For this review, take the finished solid that the model builds, in its own axes (mm). Round coordinates to 2 decimals unless told otherwise and drop trailing zeros. Loops run counter-clockwise (first coordinate to the right, second up) from the corner with the lowest first, then second, coordinate; pieces in that order, holes last. Notation, with made-up numbers: (75.5, -1) -> (107.5, -1) arc R10 ccw to (107.5, 6) -> close; hole circle Ø5 at (-15.5, 34.5). An arc over 180 degrees is marked (long way). Write each question's results on one line, items separated by ' | '.
```python
from build123d import *

# Parameters (mm, degrees)
SKETCH1_W           = 47.625
SKETCH1_H           = 152.4
SKETCH1_R           = 14.2875
BOSS_EXTRUDE1_DEPTH = 6.35
CUT_EXTRUDE1_DEPTH  = 81.086188923
FILLET1_R           = 2.54


with BuildPart() as part:
    # Sketch1 → Boss-Extrude1 (new body)
    with BuildSketch(Plane(origin=(0, 0, 0), x_dir=(1, 0, 0), z_dir=(0, 1, 0))):
        Rectangle(SKETCH1_W, SKETCH1_H)
        with Locations(Location((0, 38.1, 0), (0, 0, 270))):
            Circle(SKETCH1_R, mode=Mode.SUBTRACT)
        with Locations(Location((0, -46.99, 0), (0, 0, 270))):
            Circle(SKETCH1_R, mode=Mode.SUBTRACT)
    extrude(amount=BOSS_EXTRUDE1_DEPTH)

    # Sketch2 → Cut-Extrude1 (cut, through all)
    with BuildSketch(Plane(origin=(0, 6.35, 0), x_dir=(1, 0, 0), z_dir=(0, 1, 0))):
        with BuildLine():
            ThreePointArc((23.8125, -46.99), (0, -70.8025), (-23.8125, -46.99))
            Line((-23.8125, -46.99), (-23.8125, -76.2))
            Line((-23.8125, -76.2), (23.8125, -76.2))
            Line((23.8125, -76.2), (23.8125, -46.99))
        make_face()
        with BuildLine():
            Line((-17.4625, 69.85), (-17.4625, 54.289386956))
            ThreePointArc((-17.4625, 54.289386956), (-10.963825458, 59.238346377), (-3.175, 61.699884136))
            Line((-3.175, 61.699884136), (-3.175, 69.85))
            Line((-3.175, 69.85), (-17.4625, 69.85))
        make_face()
        with BuildLine():
            ThreePointArc((-3.175, 14.500115864), (-10.963825458, 16.961653623), (-17.4625, 21.910613044))
            Line((-17.4625, 21.910613044), (-17.4625, -30.800613044))
            ThreePointArc((-17.4625, -30.800613044), (-10.963825458, -25.851653623), (-3.175, -23.390115864))
            Line((-3.175, -23.390115864), (-3.175, 14.500115864))
        make_face()
        with BuildLine():
            ThreePointArc((3.175, 61.699884136), (10.963825458, 59.238346377), (17.4625, 54.289386956))
            Line((17.4625, 54.289386956), (17.4625, 69.85))
            Line((17.4625, 69.85), (3.175, 69.85))
            Line((3.175, 69.85), (3.175, 61.699884136))
        make_face()
        with BuildLine():
            Line((17.4625, -30.800613044), (17.4625, 21.910613044))
            ThreePointArc((17.4625, 21.910613044), (10.963825458, 16.961653623), (3.175, 14.500115864))
            Line((3.175, 14.500115864), (3.175, -23.390115864))
            ThreePointArc((3.175, -23.390115864), (10.963825458, -25.851653623), (17.4625, -30.800613044))
        make_face()
    extrude(amount=-CUT_EXTRUDE1_DEPTH, mode=Mode.SUBTRACT)

    # Fillet1
    fillet1_edges = [part.edges().sort_by_distance(p)[0] for p in [
        (17.4625, 3.175, 30.800613044),
        (3.175, 3.175, 23.390115864),
        (3.175, 3.175, -14.500115864),
        (17.4625, 3.175, -21.910613044),
        (-3.175, 3.175, 23.390115864),
        (-17.4625, 3.175, 30.800613044),
        (-17.4625, 3.175, -21.910613044),
        (-3.175, 3.175, -14.500115864),
        (-3.175, 3.175, -61.699884136),
        (-17.4625, 3.175, -54.289386956),
        (-17.4625, 3.175, -69.85),
        (-3.175, 3.175, -69.85),
        (17.4625, 3.175, -54.289386956),
        (3.175, 3.175, -61.699884136),
        (3.175, 3.175, -69.85),
        (17.4625, 3.175, -69.85),
    ]]
    fillet(fillet1_edges, radius=FILLET1_R)


solid = part.part
```
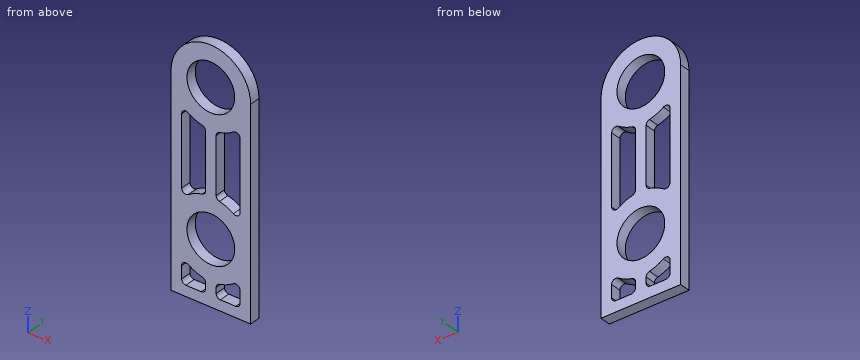
1. Consider section A-A (x = 0). State the section outline as (y, z) points.
Values found:
outline: (0, -76.2) -> (6.35, -76.2) -> (6.35, -52.39) -> (0, -52.39) -> close; (0, -23.81) -> (6.35, -23.81) -> (6.35, 32.7) -> (0, 32.7) -> close; (0, 61.28) -> (6.35, 61.28) -> (6.35, 70.8) -> (0, 70.8) -> close
2. Consider section B-B (z = -38.1). State the section outline as (x, y) points, plus the area to 3 significant figures.
Values found:
outline: (-23.81, 0) -> (-14.29, 0) -> (-14.29, 6.35) -> (-23.81, 6.35) -> close; (14.29, 0) -> (23.81, 0) -> (23.81, 6.35) -> (14.29, 6.35) -> close | area: 121 mm2
3. To check wall thickness, follow probe 1 along X at (y, z) = (4, 6) (1 decimal); probe 2 along Z at (x, y) = (12, 4); probe 3 along Z at (x, y) = (-4.5, 2.5). State the ranges of each line that lie inside material, in increasing order.
Values found:
probe 1: x = -23.8 to -17.5, -3.2 to 3.2, 17.5 to 23.8 | probe 2: z = -76.2 to -69.85, -58.67 to -45.85, -30.35 to -17.53, 26.42 to 39.24, 54.74 to 67.56 | probe 3: z = -76.2 to -69.54, -61.59 to -51.66, -24.54 to -14.61, 23.5 to 33.43, 60.55 to 70.37
4. Consider section D-D (x = 7.5). State the section outline as (y, z) points.
Values found:
outline: (0, -76.2) -> (6.35, -76.2) -> (6.35, -69.85) -> (0, -69.85) -> close; (0, -60.7) -> (6.35, -60.7) -> (6.35, -50.26) -> (0, -50.26) -> close; (0, -25.94) -> (6.35, -25.94) -> (6.35, -15.5) -> (0, -15.5) -> close; (0, 24.39) -> (6.35, 24.39) -> (6.35, 34.83) -> (0, 34.83) -> close; (0, 59.15) -> (6.35, 59.15) -> (6.35, 69.59) -> (0, 69.59) -> close
5. For pin 1 (1.9 mm diameter, centred on x = -11, y = 4.5, fed in from +Z), flat-tipped, find the tip position at first contact; note if it passes through.
Values found:
pin 1: stops at z = 68.58
6. Consider section C-C (z = -7). Give the number of separate pieces and of enclosed holes in the cut face, plus the area to 3 significant figures.
Values found:
separate pieces: 3 | enclosed holes: 0 | area: 121 mm2
